Part model, mm, in its own coordinate system. Face numbers are marked on the shaded views. A direction names the side the tool comes from. Give positions to 0.01 mm unless a question says otherwise; leave off trailing zeros. Order: outer loops, then holes, each group sorted by start corner. A loop starts at its lowest first (then second) coordinate and runs counter-clockwise, first axis right, second up. Notation, with made-up numbers: (66, 84.5) -> (76, 84.5) arc R28 ccw to (76, 119.5) -> close; hole circle Ø6 at (3.5, -22). An arc over 180 degrees is marked (long way). Write item = value, one per line. Start each with the question number.
(1) Saw through at C-C, the plane z = 40. List the corners of the cut face in (x, y), then the cut area to 3 significant figures.
(2) Probe line 1 along Y through (x, z) = (116, 40); line 2 along Z through (x, y) = (114, 160); line 3 along X through (y, z) = (6, 40). List the from-to ranges inside material, lowest first. Write a range as from..to.
(3) Which spindle directions (+Z, -Z, +X, -X, +Y, -Y) get a long thin tool onto all of the face, cutting with end or side? Do the marked faces 5 and 6. Say none if no direction does.
(4) Saw through at B-B, the plane x = 34. List the corners of the cut face in (y, z).
(5) Two-plate mould, pull along X, no slides. Class the marked faces 1, 2, 3 and 4: pulls with the +X half, pulls with the -X half, needs draft (parallel to the pull), parting line crosses it, or undercut.
(6) Saw through at A-A, the plane x = 75. List the corners of the cut face in (y, z).
(7) Saw through at D-D, the plane y = 125. List the corners of the cut face in (x, z).
(8) Flat gauge pins, fed straight in: pin 1 (13 mm diameter, centred on y = 160, z = 40, fed in from -X); pin 2 (6 mm diameter, centred on x = 122.5, z = 67.5, fed in from +Y); pin 3 (5 mm diameter, centred on y = 160, z = 39, fed in from -X). Where does each tip first touch, or does it go through?
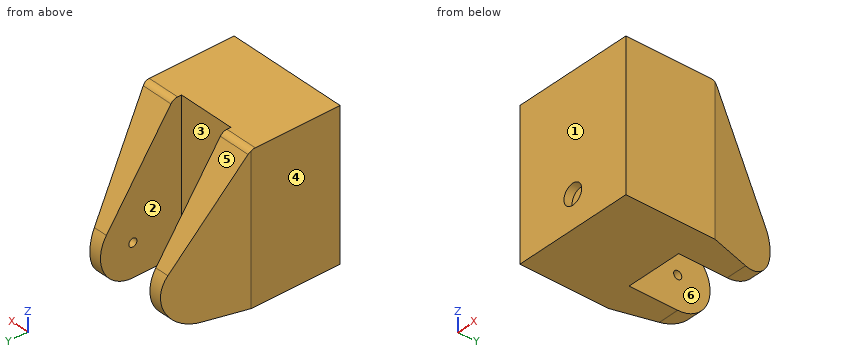
from build123d import *

# Parameters (mm, degrees)
EXTRUDE_1_DEPTH         = 150
FILLET_1_R              = 10
CUT_EXTRUDE_1_DEPTH     = 309.058436015
SKETCH1_R               = 12.5
CUT_EXTRUDE1_DEPTH      = 10
CUT_EXTRUDE2_DEPTH      = 80
CUT_EXTRUDE2_DEPTH_BACK = 10
SKETCH2_R               = 5


with BuildPart() as part:
    # 草圖1 → 填料-伸長1 (new body)
    with BuildSketch(Plane(origin=(0, 0, 0), x_dir=(0, 0, -1), z_dir=(1, 0, 0))):
        with BuildLine():
            Line((0, 0), (0, 160))
            ThreePointArc((0, 160), (-21.611444176, 195.522683101), (-63.093050736, 192.660542061))
            Line((-63.093050736, 192.660542061), (-180, 110))
            Line((-180, 110), (-180, 0))
            Line((-180, 0), (0, 0))
        make_face()
    extrude(amount=EXTRUDE_1_DEPTH)

    # 圓角1
    fillet_1_edges = [part.edges().sort_by_distance(p)[0] for p in [
        (75, 110, 180),
    ]]
    fillet(fillet_1_edges, radius=FILLET_1_R)

    # 草圖2 → 除料-伸長1 (cut, through all)
    with BuildSketch(Plane(origin=(0, 0, 0), x_dir=(-1, 0, 0), z_dir=(0, 0, -1))):
        Polygon((-150, 110), (-125, 200), (-125, 212.317241835), (-176.077029544, 212.317241835), (-176.077029544, 111.407234288), align=None)
        Polygon((-110, 110), (-110, 202.916849344), (-40, 202.916849344), (-40, 110), (-40, 100), (-110, 100), align=None)
        Polygon((26.077029544, 111.407234288), (0, 110), (-25, 200), (-25, 212.317241835), (26.077029544, 212.317241835), align=None)
    extrude(amount=-CUT_EXTRUDE_1_DEPTH, mode=Mode.SUBTRACT)

    # Sketch1 → Cut-Extrude1 (cut)
    with BuildSketch(Plane.XZ):
        with Locations(Location((75, 40, 0), (0, 0, 270))):
            Circle(SKETCH1_R)
    extrude(amount=-CUT_EXTRUDE1_DEPTH, mode=Mode.SUBTRACT)

    # Sketch2 → Cut-Extrude2 (cut, two sides: drawn at the far end of the back side and taken through both)
    with BuildSketch(Plane(origin=(40, 0, 0), x_dir=(0, 0, -1), z_dir=(1, 0, 0)).offset(-CUT_EXTRUDE2_DEPTH_BACK)):
        with Locations(Location((-40, 160, 0), (0, 0, 270))):
            Circle(SKETCH2_R)
    extrude(amount=CUT_EXTRUDE2_DEPTH + CUT_EXTRUDE2_DEPTH_BACK, mode=Mode.SUBTRACT)


solid = part.part
Results list:
q1.outline = (0, 0) -> (62.5, 0) -> (62.5, 10) -> (87.5, 10) -> (87.5, 0) -> (150, 0) -> (150, 110) -> (125, 200) -> (110, 200) -> (110, 165) -> (120, 165) -> (120, 155) -> (110, 155) -> (110, 100) -> (40, 100) -> (40, 155) -> (30, 155) -> (30, 165) -> (40, 165) -> (40, 200) -> (25, 200) -> (0, 110) -> close
q1.area = 20,300 mm^2
q2.line_1 = 0..155, 165..200
q2.line_2 = 0..35, 45..109.28
q2.line_3 = 0..62.5, 87.5..150
q3.face_5 = +Z, +X, -X, +Y
q3.face_6 = +Z, -Z, +Y
q4.outline = (0, 0) -> (160, 0) arc R40 ccw to (192.66, 63.09) -> (112.99, 175.77) arc R10 ccw to (104.82, 180) -> (0, 180) -> close; hole circle Ø10 at (160, 40)
q5.face_1 = needs draft
q5.face_2 = undercut
q5.face_3 = undercut
q5.face_4 = pulls with the -X half
q6.outline = (0, 0) -> (100, 0) -> (100, 180) -> (0, 180) -> (0, 52.5) -> (10, 52.5) -> (10, 27.5) -> (0, 27.5) -> close
q7.outline = (4.17, 0) -> (40, 0) -> (40, 158.79) -> (4.17, 158.79) -> close; (110, 0) -> (145.83, 0) -> (145.83, 158.79) -> (110, 158.79) -> close
q8.pin_1 = 12.08
q8.pin_2 = 191.67
q8.pin_3 = 13.19
